Read the model definition and answer for the solid it produces. Units are mm, in the model's axes. A direction names the side the tool comes from. Coordinates: 2 decimals unless noted, no trailing zeros. Write each loop counter-clockwise with the first axis right and the second up, starting at its lowest first coordinate (ties: lowest second). Pieces come first, ordered by that corner, then holes.
Item 1: Section B-B (x = -28) is taken. Give the vertices of the cut face in (y, z) (3 decimals).
Item 2: Section D-D (y = 12.25) is taken. State how many separate pieces and enclosed holes the cut face has, then the cut area to 3 significant figures.
Item 3: Section C-C (x = -11) is taken. Give the vertices of the cut face in (y, z) (3 decimals), then the cut area to 3 significant figures.
Item 4: A tool of negligible diameter and unlimited length cuts with its end or side. For faces 5 (the face through (9.1, 21, 0)), 6 (the face through (21, 14, -16)), 7 (the face through (-17.075, 13.478, 0.245)), from which of +Z, -Z, +X, -X, +Y, -Y can it reach the whole face along a straight path? Write none if from no direction.
Item 5: Determine the mould class of faces 1 (the face through (20, 13, -20.5)), 2 (the face through (-37.719, 2.406, -0.035)), 3 (the face through (-6, 22, 22.5)), 4 (the face through (22.778, 11.321, -18.688)) for opening direction X: released by +X, released by -X, zero draft, split by the parting line, or undercut.
Item 6: Straight lines are drawn through the part: probe 1 along X at (y, z) = (21, -17.5); probe 2 along X at (y, z) = (18.5, 17.5); probe 3 along X at (y, z) = (16.5, 17.5). For each, find the intervals that lie inside material, in ascending order.
Item 7: Section A-A (x = -20) is taken. Give the vertices of the cut face in (y, z) (3 decimals).
Item 8: Each of these flat-tipped pins is pushed along its axis until it touches: P1, Ø0.8, axis at x = -20, y = 12.5, coming from the -Z side; P2, Ø1, axis at x = -19, y = 11, coming from the +Z side; P3, Ø6, axis at x = 25.5, z = 1.5, coming from the +Y side. Where does it stop, or does it pass through?
from build123d import *

# Parameters (mm, degrees)
SKETCH1_W           = 80
SKETCH1_H           = 45
BOSS_EXTRUDE1_DEPTH = 24.6
SKETCH3_W           = 30
SKETCH3_H           = 12.15
CUT_EXTRUDE1_DEPTH  = 5.1
SKETCH4_R           = 4.05
CUT_EXTRUDE2_DEPTH  = 66.039680196
SKETCH5_R           = 1.5
CUT_EXTRUDE3_DEPTH  = 31
FILLET1_START       = -40
FILLET1_DEPTH       = 80
FILLET2_R           = 20
CUT_EXTRUDE4_DEPTH  = 14
FILLET3_R           = 8


with BuildPart() as part:
    # Sketch1 → Boss-Extrude1 (new body)
    with BuildSketch(Plane(origin=(0, 0, 0), x_dir=(1, 0, 0), z_dir=(0, 1, 0))):
        Rectangle(SKETCH1_W, SKETCH1_H)
    extrude(amount=BOSS_EXTRUDE1_DEPTH)

    # Sketch2 → Cut-Revolve1 (revolve, cut)
    with BuildSketch(Plane(origin=(0, 24.6, 0), x_dir=(1, 0, 0), z_dir=(0, 1, 0))):
        Polygon((8.5, 3.125), (9.5, 3.125), (9.5, 0), (6, 0), (-40, 0), (-40, 11.125), (-37, 11.125), (-37, 16.125), (-29.75, 16.125), (-29.75, 11.125), (-4.75, 11.125), (-4.75, 16.125), (2.5, 16.125), (2.5, 11.125), (8.5, 11.125), align=None)
    revolve(axis=Axis((-40, 24.6, 0), (1, 0, 0)), mode=Mode.SUBTRACT)

    # Sketch3 → Cut-Extrude1 (cut)
    with BuildSketch(Plane(origin=(0, 24.6, 0), x_dir=(1, 0, 0), z_dir=(0, 1, 0))):
        with Locations((24.1, 0)):
            Rectangle(SKETCH3_W, SKETCH3_H)
    extrude(amount=-CUT_EXTRUDE1_DEPTH, mode=Mode.SUBTRACT)

    # Sketch4 → Cut-Extrude2 (cut, through all)
    with BuildSketch(Plane.XY.offset(22.5)):
        with Locations((-11, 24.6)):
            Circle(SKETCH4_R)
    extrude(amount=-CUT_EXTRUDE2_DEPTH, mode=Mode.SUBTRACT)

    # Sketch5 → Cut-Extrude3 (cut)
    with BuildSketch(Plane(origin=(0, 24.6, 0), x_dir=(1, 0, 0), z_dir=(0, 1, 0))):
        with Locations(Location((-20, 17.5, 0), (0, 0, 270))):
            Circle(SKETCH5_R)
        with Locations(Location((-20, -17.5, 0), (0, 0, 270))):
            Circle(SKETCH5_R)
        with Locations(Location((20, -17.5, 0), (0, 0, 270))):
            Circle(SKETCH5_R)
        with Locations(Location((20, 17.5, 0), (0, 0, 270))):
            Circle(SKETCH5_R)
    extrude(amount=-CUT_EXTRUDE3_DEPTH, mode=Mode.SUBTRACT)

    # Fillet1: read off the stored shape, not the designer's step
    # Fillet1 outline → Fillet1 (cut)
    with BuildSketch(Plane.YZ.offset(FILLET1_START)):
        with BuildLine():
            Line((0, 22.5), (0, 2.5))
            ThreePointArc((0, 2.5), (5.857864376, 16.642135624), (20, 22.5))
            Line((20, 22.5), (0, 22.5))
        make_face()
        with BuildLine():
            ThreePointArc((20, -22.5), (5.857864376, -16.642135624), (0, -2.5))
            Line((0, -2.5), (0, -22.5))
            Line((0, -22.5), (20, -22.5))
        make_face()
    extrude(amount=FILLET1_DEPTH, mode=Mode.SUBTRACT)

    # Fillet2
    # the kernel refuses this fillet: 20 mm, written as the material it takes off along each edge
    with BuildSketch(Plane(origin=(40, 0, 2.5), x_dir=(0, 1, 0), z_dir=(0, 0, -1))) as fillet2_piece_1:
        with BuildLine():
            CenterArc((FILLET2_R, -FILLET2_R), FILLET2_R, 90, 90)
            Line((0, -FILLET2_R), (0, 0))
            Line((0, 0), (FILLET2_R, 0))
        make_face()
    extrude(amount=5, mode=Mode.SUBTRACT)
    with BuildSketch(Plane(origin=(40, 19.999999999, 2.500000001), x_dir=(0, -1.0, -4.592977109962882e-11), z_dir=(0, 4.592977109962882e-11, -1.0))) as fillet2_piece_2:
        with BuildLine():
            CenterArc((19.999999999 - FILLET2_R, FILLET2_R), FILLET2_R, 270, 90)
            Line((19.999999999 - FILLET2_R, 0), (19.999999999, 0))
            Line((19.999999999, 0), (19.999999999, FILLET2_R))
        make_face()
    revolve(axis=Axis((40, 19.999999999, 2.500000001), (-1, 0, 0)), revolution_arc=90.000000005, mode=Mode.SUBTRACT)
    with BuildSketch(Plane(origin=(40, 19.999999999, -2.500000001), x_dir=(0, 4.592966007732635e-11, -1.0), z_dir=(0, 1.0, 4.592966007732635e-11))) as fillet2_piece_3:
        with BuildLine():
            CenterArc((19.999999999 - FILLET2_R, FILLET2_R), FILLET2_R, 270, 90)
            Line((19.999999999, FILLET2_R), (19.999999999, 0))
            Line((19.999999999, 0), (19.999999999 - FILLET2_R, 0))
        make_face()
    revolve(axis=Axis((40, 19.999999999, -2.500000001), (-1, 0, 0)), revolution_arc=90.000000005, mode=Mode.SUBTRACT)
    with BuildSketch(Plane(origin=(40, 20, 22.5), x_dir=(-1, 0, 0), z_dir=(0, 1, 0)), Plane(origin=(40, 20, -22.5), x_dir=(0, 0, 1), z_dir=(0, 1, 0))) as fillet2_piece_4:
        with BuildLine():
            CenterArc((FILLET2_R, -FILLET2_R), FILLET2_R, 90, 90)
            Line((0, -FILLET2_R), (0, 0))
            Line((0, 0), (FILLET2_R, 0))
        make_face()
    extrude(amount=54.6, mode=Mode.SUBTRACT)

    # Sketch6 → Cut-Extrude4 (cut)
    with BuildSketch(Plane.XZ):
        Polygon((21.732050808, 20.5), (18.267949192, 20.5), (16.535898385, 17.5), (18.267949192, 14.5), (21.732050808, 14.5), (23.464101615, 17.5), align=None)
        Polygon((-18.267949192, 20.5), (-21.732050808, 20.5), (-23.464101615, 17.5), (-21.732050808, 14.5), (-18.267949192, 14.5), (-16.535898385, 17.5), align=None)
        Polygon((-18.267949192, -14.5), (-21.732050808, -14.5), (-23.464101615, -17.5), (-21.732050808, -20.5), (-18.267949192, -20.5), (-16.535898385, -17.5), align=None)
        Polygon((21.732050808, -14.5), (18.267949192, -14.5), (16.535898385, -17.5), (18.267949192, -20.5), (21.732050808, -20.5), (23.464101615, -17.5), align=None)
    extrude(amount=-CUT_EXTRUDE4_DEPTH, mode=Mode.SUBTRACT)

    # Fillet3
    fillet3_edges = [part.edges().sort_by_distance(p)[0] for p in [
        (-40, 0, 0),
        (-40, 5.857864376, 16.642135624),
        (-40, 5.857864376, -16.642135624),
        (-40, 22.3, 22.5),
        (-40, 22.3, -22.5),
    ]]
    fillet(fillet3_edges, radius=FILLET3_R)


solid = part.part
Established:
1. outline: (0, -2.5) arc R20 ccw to (20, -22.5) - (24.6, -22.5) - (24.6, -11.125) arc R11.125 cw to (24.6, 11.125) - (24.6, 22.5) - (20, 22.5) arc R20 ccw to (0, 2.5) - close
2. separate pieces: 1
2. enclosed holes: 6
2. area: 2,680 mm2
3. outline: (0, -2.5) arc R20 ccw to (20, -22.5) - (20.55, -22.5) - (20.55, -10.362) arc R11.125 cw to (20.55, 10.362) - (20.55, 22.5) - (20, 22.5) arc R20 ccw to (0, 2.5) - close
3. area: 647 mm2
4. face 5: +Y
4. face 6: -Y
4. face 7: -X, +Y
5. face 1: undercut
5. face 2: released by -X
5. face 3: zero draft
5. face 4: undercut
6. probe 1: x = -39.42 to -21.5, -18.5 to -12.86, -9.14 to 18.5, 21.5 to 33.23
6. probe 2: x = -39.39 to -21.5, -18.5 to 18.5, 21.5 to 33.14
6. probe 3: x = -39.24 to -21.5, -18.5 to 18.5, 21.5 to 32.76
7. outline: (0, -2.5) arc R20 ccw to (4, -14.5) - (14, -14.5) - (14, -16) - (24.6, -16) - (24.6, -11.125) arc R11.125 cw to (24.6, 11.125) - (24.6, 16) - (14, 16) - (14, 14.5) - (4, 14.5) arc R20 ccw to (0, 2.5) - close; (11.282, -20.5) arc R20 ccw to (20, -22.5) - (24.6, -22.5) - (24.6, -19) - (14, -19) - (14, -20.5) - close; (11.282, 20.5) - (14, 20.5) - (14, 19) - (24.6, 19) - (24.6, 22.5) - (20, 22.5) arc R20 ccw to start
8. P1: stops at z = -21.2
8. P2: stops at z = 20.6
8. P3: stops at y = 19.5
